Work out the finished part from the listing and answer in its coordinate system (mm). Face numbers are marked on the shaded views. Coordinates: 2 decimals unless noted, no trailing zeros. Order: outer loops, then holes, each group sorted by start corner. A loop starts at its lowest first (then second) coordinate and runs counter-clockwise, first axis right, second up. Notation, with made-up numbers: M -8,-23 L 46,-23 A34 cw 46,8 Z; hole C -15.5,33.25 d9. An arc over 180 degrees is marked long. Use a Markdown table: item, result.
from build123d import *

# Parameters (mm, degrees)
F0_W        = 50.8
F0_H        = 25.4
F0_W_2      = 44.45
F0_H_2      = 19.05
F0_R        = 2.38125
F1_DEPTH    = 0.79375
F2_DEPTH    = 1.5875
F3_R        = 4.7625
F4_T1_DEPTH = 25.4
F4_T3_DEPTH = 54.9118947857
F4_T5_DEPTH = 29.5118947857
F4_T8_ANGLE = 90
F5_T1_DEPTH = 39.6011909767


# Not quite as in the source:
# - a fillet or chamfer that OpenCascade refuses, or shapes differently, is made with other operations: its cross-section is extruded or revolved along the edge and cut away or added


with BuildPart() as f1:
    # F0 (on Top) → F1 (new body)
    with BuildSketch(Plane.XY):
        with Locations((25.4, 12.7)):
            Rectangle(F0_W, F0_H)
        with Locations((25.4, 12.7)):
            Rectangle(F0_W_2, F0_H_2, mode=Mode.SUBTRACT)
        with Locations((25.4, 12.7)):
            Rectangle(F0_W_2, F0_H_2)
        with Locations((7.14375, 12.7)):
            Circle(F0_R, mode=Mode.SUBTRACT)
    extrude(amount=F1_DEPTH)

    # F0 (on Top) → F2 (join)
    with BuildSketch(Plane.XY):
        with Locations((25.4, 12.7)):
            Rectangle(F0_W, F0_H)
        with Locations((25.4, 12.7)):
            Rectangle(F0_W_2, F0_H_2, mode=Mode.SUBTRACT)
    extrude(amount=F2_DEPTH)

    # F3
    f3_edges = [f1.edges().sort_by_distance(p)[0] for p in [
        (50.8, 0, 0.79375),
    ]]
    fillet(f3_edges, radius=F3_R)

    # F4: fillet of radius 4.7625 on 2 edges, made by hand

    # F4_s2 → F4_t1 (cut)
    with BuildSketch(Plane.XY.offset(-11.90625)):
        with BuildLine():
            ThreePointArc((50.8, 20.6375), (49.4050960454, 24.0050960454), (46.0375, 25.4))
            Line((46.0375, 25.4), (50.8, 25.4))
            Line((50.8, 25.4), (50.8, 20.6375))
        make_face()
    extrude(amount=F4_T1_DEPTH, mode=Mode.SUBTRACT)

    # F4_s4 → F4_t3 (cut)
    with BuildSketch(Plane.YZ.offset(-8.8743947857)):
        with BuildLine():
            ThreePointArc((3.5497579143, 1.5875), (1.6054754309, 1.1725478002), (0, 0))
            Line((0, 0), (0, 1.5875))
            Line((0, 1.5875), (3.5497579143, 1.5875))
        make_face()
    extrude(amount=F4_T3_DEPTH, mode=Mode.SUBTRACT)

    # F4_s6 → F4_t5 (cut)
    with BuildSketch(Plane.XZ.offset(-34.2743947857)):
        with BuildLine():
            ThreePointArc((47.2502420857, 1.5875), (49.1945245691, 1.1725478002), (50.8, 0))
            Line((50.8, 0), (50.8, 1.5875))
            Line((50.8, 1.5875), (47.2502420857, 1.5875))
        make_face()
    extrude(amount=F4_T5_DEPTH, mode=Mode.SUBTRACT)

    # F4_s7 → F4_t8 (revolve, cut)
    with BuildSketch(Plane.XZ.offset(-4.7625)):
        with BuildLine():
            ThreePointArc((47.2502420857, 1.5875), (49.1945245691, 1.1725478002), (50.8, 0))
            Line((50.8, 0), (50.8, 1.5875))
            Line((50.8, 1.5875), (47.2502420857, 1.5875))
        make_face()
    revolve(axis=Axis((46.0375, 4.7625, 1.5875), (0, 0, -1)), revolution_arc=F4_T8_ANGLE, mode=Mode.SUBTRACT)

    # F5: fillet of radius 4.7625 on 1 edges, made by hand

    # F5_s2 → F5_t1 (cut)
    with BuildSketch(Plane.XZ.offset(-34.2754744455)):
        with BuildLine():
            ThreePointArc((-0.0002981182, 0.0002666937), (1.6055468798, 1.1729169704), (3.5501897557, 1.5879))
            Line((3.5501897557, 1.5879), (3.5501897557, 2.0642865685))
            ThreePointArc((3.5501897557, 2.0642865685), (1.7750948778, 2.0638865685), (0, 2.0638865685))
            Line((0, 2.0638865685), (-0.4763865685, 1.5875))
            ThreePointArc((-0.4763865685, 1.5875), (-0.4763865685, 0.7938833468), (-0.3553469056, 0.3178899316))
            Line((-0.3553469056, 0.3178899316), (-0.0002981182, 0.0002666937))
        make_face()
    extrude(amount=F5_T1_DEPTH, mode=Mode.SUBTRACT)


solid = f1.part
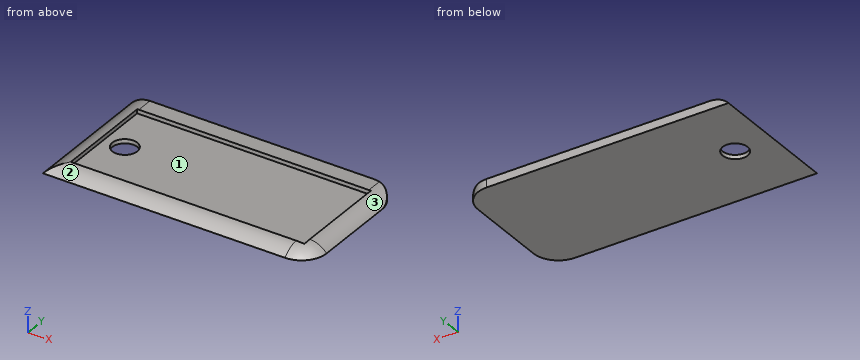
1. For a pull along X with two mould halves and no side action, classify the marked faces 1, 2 and 3 as +X half, -X half, draft (parallel to the pull), parting line (faces both ways), or undercut.
Answers below:
| item | result |
|---|---|
| face 1 | undercut |
| face 2 | draft |
| face 3 | +X half |
2. Flat-ended cylindrical pins translate along their axes: P1, Ø0.9, axis at y = 12.5, z = 1, coming from the +X side; P2, Ø3, axis at x = 14, y = 18, coming from the +Z side. Find the tip coordinate at first contact, or state that the pin passes through.
Answers below:
| item | result |
|---|---|
| P1 | x = 50.22 |
| P2 | z = 0.79 |
3. Section B-B on x = 39.5 is taken. Determine the outline of the cut face in (y, z) (1 decimal).
Answers below:
| item | result |
|---|---|
| outline | M 0,0 L 25.4,0 L 25.4,1.6 L 22.2,1.6 L 22.2,0.8 L 3.2,0.8 L 3.2,1.6 A4.8 ccw Z |
4. Find the intervals of material crossed by probe 1 along Z at (x, y) = (45, 12); probe 2 along X at (y, z) = (17.75, 1.05) (3 decimals); probe 3 along X at (y, z) = (14.25, 1.15) (3 decimals), in increasing order.
Answers below:
| item | result |
|---|---|
| probe 1 | 0 to 0.79 |
| probe 2 | 1.351 to 3.175, 47.625 to 49.448 |
| probe 3 | 1.555 to 3.175, 47.625 to 49.244 |
